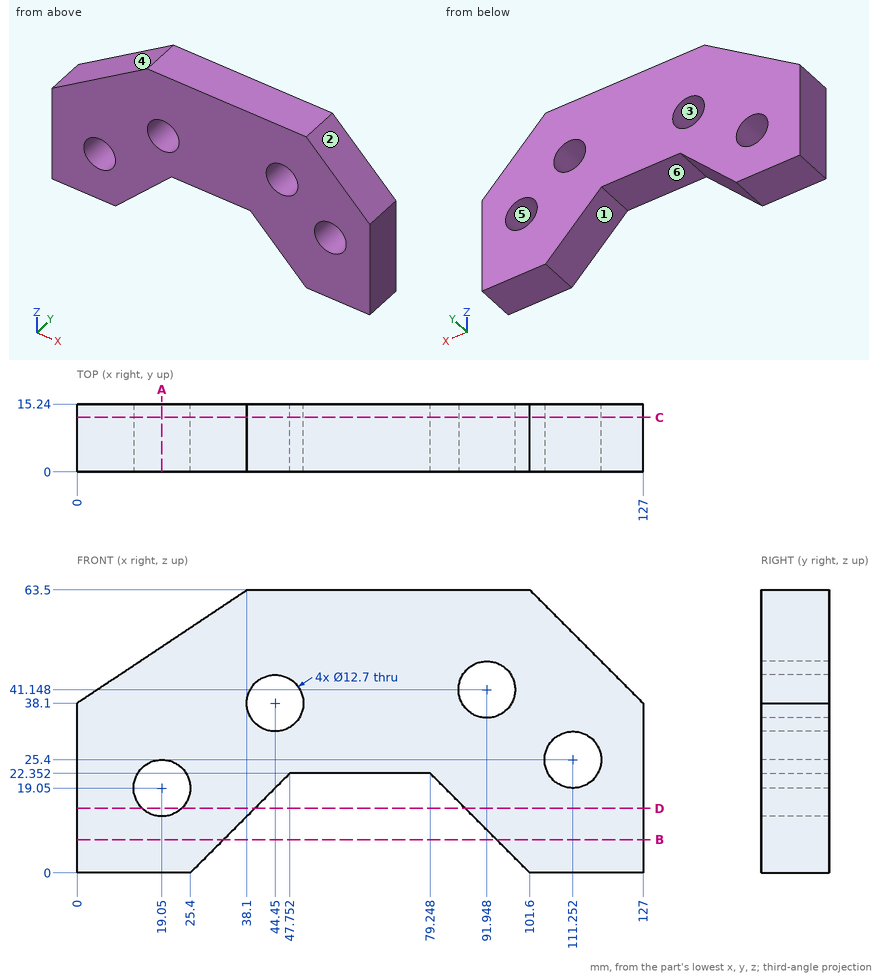
Geometry check sheet. Reference: drawing and pictorial views, mm from the part's lowest x, y, z. A direction names the side the tool comes from. Round coordinates to 2 decimals unless told otherwise and drop trailing zeros. Loops run counter-clockwise (first coordinate to the right, second up) from the corner with the lowest first, then second, coordinate; pieces in that order, holes last.
1. Sectioned sample at B-B on z = 7.5. Record the boundary of the cut face in (x, y), and give its area (3 significant figures).
2. Mould release check, pull along Z, two halves, no side actions. Record for the marked faces 3, 4, 5 and 6: released by +Z, released by -Z, zero draft, split by the parting line, or undercut.
3. Scan lines: probe 1 along Z at (x, y) = (44.45, 9.75); probe 2 along Z at (x, y) = (19.05, 6.5); probe 3 along X at (y, z) = (13.75, 36). Record each from-to range of solid material in increasing order.
4. Sectioned sample at A-A on x = 19.05. Record the boundary of the cut face in (y, z).
5. Sectioned sample at C-C on y = 12.25. Record the boundary of the cut face in (x, z).
6. Set-up check for the marked faces 1 and 2: record each of +Z, -Z, +X, -X, +Y, -Y from which the full face is reachable in a straight line by a thin tool's end or side.
7. Gauge pin test, flat ends, axial feed: pin 1 Ø20.5 at (x, z) = (111.252, 25.4) entering from -Y; pin 2 Ø8 at (x, y) = (44.5, 11) entering from -Z; pin 3 Ø3 at (x, y) = (38, 9.5) entering from -Z; pin 4 Ø8 at (x, z) = (90.5, 40) entering from -Y. Record the tip position at first contact, or that the pin passes through.
8. Sectioned sample at D-D on z = 14.5. Record the boundary of the cut face in (x, y), and give its area (3 significant figures).
Recorded:
1. outline: (0, 0) - (32.9, 0) - (32.9, 15.24) - (0, 15.24) - close; (94.1, 0) - (127, 0) - (127, 15.24) - (94.1, 15.24) - close
1. area: 1,000 mm2
2. face 3: undercut
2. face 4: released by +Z
2. face 5: undercut
2. face 6: released by -Z
3. probe 1: z = 19.05 to 31.75, 44.45 to 63.5
3. probe 2: z = 0 to 12.7, 25.4 to 50.8
3. probe 3: x = 0 to 38.46, 50.44 to 88.23, 95.67 to 127
4. outline: (0, 0) - (15.24, 0) - (15.24, 12.7) - (0, 12.7) - close; (0, 25.4) - (15.24, 25.4) - (15.24, 50.8) - (0, 50.8) - close
5. outline: (0, 0) - (25.4, 0) - (47.75, 22.35) - (79.25, 22.35) - (101.6, 0) - (127, 0) - (127, 38.1) - (101.6, 63.5) - (38.1, 63.5) - (0, 38.1) - close; hole circle Ø12.7 at (19.05, 19.05); hole circle Ø12.7 at (44.45, 38.1); hole circle Ø12.7 at (91.95, 41.15); hole circle Ø12.7 at (111.25, 25.4)
6. face 1: -Z, +Y, -Y
6. face 2: +Z, +X, +Y, -Y
7. pin 1: stops at y = 0
7. pin 2: stops at z = 15.1
7. pin 3: stops at z = 11.1
7. pin 4: passes through
8. outline: (0, 0) - (14.62, 0) - (14.62, 15.24) - (0, 15.24) - close; (23.48, 0) - (39.9, 0) - (39.9, 15.24) - (23.48, 15.24) - close; (87.1, 0) - (127, 0) - (127, 15.24) - (87.1, 15.24) - close
8. area: 1,080 mm2
